Can you work these out from the model? Positions are in its coordinate system, mm. A direction names the side the tool comes from. Give positions to 0.01 mm unless a question says otherwise; leave off trailing zeros. Write each loop counter-clockwise with the first axis right and the second up, starting at its lowest first coordinate (ties: lowest second). Pieces come first, ordered by that corner, then holes. Notation, with made-up numbers: M 6.25,70 L 42.25,70 A16 ccw 42.25,89 Z; hole C 31.25,-13.75 d7. An arc over 180 degrees is marked long. Write each question's results on one line, items separated by ' | '.
from build123d import *

# Parameters (mm, degrees)
F0_W     = 76.2
F0_H     = 12.7
F1_DEPTH = 25.4
F3_DEPTH = 12.7
F4_R     = 6.35
F5_DEPTH = 25.4


# Not quite as in the source:
# - ends of sketch curves that miss each other by under 0.0002 mm in the source are joined


with BuildPart() as f1:
    # F0 (on Front) → F1 (new body)
    with BuildSketch(Plane.XZ):
        with Locations((38.1, 6.35)):
            Rectangle(F0_W, F0_H)
    extrude(amount=F1_DEPTH)

    # F2 (on face) → F3 (cut)
    with BuildSketch(Plane.XY.offset(12.7)):
        with BuildLine():
            Line((0, -25.4), (12.7, -25.4))
            ThreePointArc((12.7, -25.4), (3.7197438789, -21.6802561211), (0, -12.7))
            Line((0, -12.7), (0, -25.4))
        make_face()
        with BuildLine():
            ThreePointArc((0, -12.7), (3.7197438789, -3.7197438789), (12.7, 0))
            Line((12.7, 0), (0, 0))
            Line((0, 0), (0, -12.7))
        make_face()
        with BuildLine():
            ThreePointArc((63.5, -19.05), (57.15, -12.7), (63.5, -6.35))
            Line((63.5, -6.35), (38.0999993506, -6.35))
            ThreePointArc((38.0999993506, -6.35), (42.5901278309, -8.2098717099), (44.45, -12.7))
            ThreePointArc((44.45, -12.7), (42.5901280605, -17.1901280605), (38.1, -19.05))
            Line((38.1, -19.05), (63.5, -19.05))
        make_face()
        with BuildLine():
            Line((38.0999996753, -12.7), (38.0999993506, -6.35))
            ThreePointArc((38.0999993506, -6.35), (33.6098717099, -8.2098721691), (31.75, -12.7))
            Line((31.75, -12.7), (38.0999996753, -12.7))
        make_face()
        with BuildLine():
            ThreePointArc((31.75, -12.7), (33.6098719395, -17.1901280605), (38.1, -19.05))
            Line((38.1, -19.05), (38.0999996753, -12.7))
            Line((38.0999996753, -12.7), (31.75, -12.7))
        make_face()
        with BuildLine():
            ThreePointArc((44.45, -12.7), (42.5901278309, -8.2098717099), (38.0999993506, -6.35))
            Line((38.0999993506, -6.35), (38.0999996753, -12.7))
            Line((38.0999996753, -12.7), (38.1, -19.05))
            ThreePointArc((38.1, -19.05), (42.5901280605, -17.1901280605), (44.45, -12.7))
        make_face()
        with BuildLine():
            Line((63.5, -19.05), (63.5, -6.35))
            ThreePointArc((63.5, -6.35), (57.15, -12.7), (63.5, -19.05))
        make_face()
        with BuildLine():
            ThreePointArc((63.5, -19.05), (67.9901280605, -17.1901280605), (69.85, -12.7))
            ThreePointArc((69.85, -12.7), (67.9901280605, -8.2098719395), (63.5, -6.35))
            Line((63.5, -6.35), (63.5, -19.05))
        make_face()
        with BuildLine():
            Line((76.2, 0), (63.5, 0))
            ThreePointArc((63.5, 0), (72.4802561211, -3.7197438789), (76.2, -12.7))
            Line((76.2, -12.7), (76.2, 0))
        make_face()
        with BuildLine():
            ThreePointArc((76.2, -12.7), (72.4802561211, -21.6802561211), (63.5, -25.4))
            Line((63.5, -25.4), (76.2, -25.4))
            Line((76.2, -25.4), (76.2, -12.7))
        make_face()
    extrude(amount=-F3_DEPTH, mode=Mode.SUBTRACT)

    # F4 (on face) → F5 (join)
    with BuildSketch(Plane.XY.offset(12.7)):
        with BuildLine():
            ThreePointArc((12.7, -25.4), (21.6802561211, -21.6802561211), (25.4, -12.7))
            ThreePointArc((25.4, -12.7), (21.6802561211, -3.7197438789), (12.7, 0))
            ThreePointArc((12.7, 0), (0, -12.7), (12.7, -25.4))
        make_face()
        with Locations((12.7, -12.7)):
            Circle(F4_R, mode=Mode.SUBTRACT)
    extrude(amount=F5_DEPTH)


solid = f1.part
Item 1: I want a section at A-A, the plane x = 54. Please give me the cut outline in (y, z), and give its area (3 significant figures).
Geometry says:
outline: M -25.4,0 L -19.05,0 L -19.05,12.7 L -25.4,12.7 Z; M -6.35,0 L 0,0 L 0,12.7 L -6.35,12.7 Z | area: 161 mm2
Item 2: I want a section at C-C, the plane y = -7.25. Please give me the cut outline in (x, z).
Geometry says:
outline: M 1.23,0 L 34.84,0 L 34.84,12.7 L 24.17,12.7 L 24.17,38.1 L 15.96,38.1 L 15.96,12.7 L 9.44,12.7 L 9.44,38.1 L 1.23,38.1 Z; M 66.76,0 L 74.97,0 L 74.97,12.7 L 66.76,12.7 Z
Item 3: I'm going to push flat-ended pins straight in: pin 1 (7.5 mm diameter, centred on x = 42.5, y = -18.5, fed in from +Z); pin 2 (4 mm diameter, centred on x = 8, z = 30.5, fed in from -Y); pin 3 (1 mm diameter, centred on y = -14.5, z = 7, fed in from -X); pin 4 (4 mm diameter, centred on x = 38, y = -8.5, fed in from -Z). Where does each tip first touch, or does it pass through?
Geometry says:
pin 1: stops at z = 12.7 | pin 2: stops at y = -25.11 | pin 3: stops at x = 0.07 | pin 4: passes through
Item 4: I want a section at D-D, the plane y = -11.25. Please give me the cut outline in (x, z).
Geometry says:
outline: M 0.08,0 L 31.92,0 L 31.92,12.7 L 25.32,12.7 L 25.32,38.1 L 18.88,38.1 L 18.88,12.7 L 6.52,12.7 L 6.52,38.1 L 0.08,38.1 Z; M 69.68,0 L 76.12,0 L 76.12,12.7 L 69.68,12.7 Z
Item 5: I want a section at B-B, the plane z = 8.5. Please give me the cut outline in (x, y).
Geometry says:
outline: M 12.7,-25.4 L 63.5,-25.4 A12.7 ccw 63.5,0 L 12.7,0 A12.7 ccw Z; hole M 38.1,-19.05 L 63.5,-19.05 A6.35 ccw 63.5,-6.35 L 38.1,-6.35 A6.35 ccw Z
Item 6: Thinking about a two-plate mould opening in Y: for faces 4 (the face through (6.9, -9.7, 38.1)), 5 (the face through (38, 0, 6)), 6 (the face through (7.66, -16.56, 25.22)), which applies, +Y half, -Y half, draft (parallel to the pull), parting line (faces both ways), or undercut?
Geometry says:
face 4: draft | face 5: +Y half | face 6: undercut
Item 7: If I drill on line 1 (Y direction, x = 12.7, z = 27); line 2 (Z direction, x = 43.5, y = -3.5); line 3 (X direction, y = -16, z = 33), over which ranges is the centre line in solid material (lowest first)? Write a range as from..to.
Geometry says:
line 1: y = -25.4..-19.05, -6.35..0 | line 2: z = 0..12.7 | line 3: x = 0.44..7.27, 18.13..24.96
Item 8: For faces 1 (the face through (29, -13, 0)), 2 (the face through (13, -13, 12.7)), 3 (the face through (51, -6.35, 6)), which set-ups out of +Z, -Z, +X, -X, +Y, -Y let a thin tool reach every point of the face, with its end or its side?
Geometry says:
face 1: -Z, +X, -X, +Y, -Y | face 2: +Z | face 3: +Z, -Z
